from build123d import *

# Parameters (mm, degrees)
EXTRUDE019_DEPTH = 20
SKETCH022_R      = 2
EXTRUDE017_DEPTH = 7.5
FILLET008_R      = 2
SKETCH021_R      = 1
EXTRUDE016_DEPTH = 5
FILLET007_R      = 2
EXTRUDE018_DEPTH = 13
EXTRUDE007_DEPTH = 20
SKETCH008_R      = 1
EXTRUDE004_DEPTH = 5
FILLET001_R      = 2
SKETCH005_R      = 11.5
EXTRUDE003_DEPTH = 2.5
FILLET_R         = 1
SKETCH006_R      = 1.625
SKETCH006_R_2    = 5.532603
EXTRUDE002_DEPTH = 6
SKETCH009_R      = 2
EXTRUDE005_DEPTH = 7.5
FILLET002_R      = 2


with BuildPart() as extrude019:
    # Sketch024 (on Face5 of Cut001) → Extrude019 (new body, symmetric)
    with BuildSketch(Plane.XY.offset(6)):
        with BuildLine():
            ThreePointArc((18.40856, 16.235038), (15.499807, 18.5), (12.591346, 16.234663))
            ThreePointArc((12.10657, 15.857107), (12.413798, 15.962631), (12.591346, 16.234663))
            Line((12.10657, 15.857107), (12.10657, 10.857107))
            Line((12.10657, 10.857107), (18.905391, 10.857107))
            Line((18.905391, 15.85769), (18.905391, 10.857107))
            ThreePointArc((18.40856, 16.235038), (18.590902, 15.959369), (18.905391, 15.85769))
        make_face()
    extrude(amount=EXTRUDE019_DEPTH, both=True)


with BuildPart() as extrude019_1:
    # Extrude019 placement: moved
    add(extrude019.part.moved(Location((-31, 0, 10))))


with BuildPart() as fillet008:
    # Sketch022 (on Face2 of Cut001) → Extrude017 (new body)
    with BuildSketch(Plane(origin=(0, 20.857107, 0), x_dir=(-1, 0, 0), z_dir=(0, 1, 0))):
        with BuildLine():
            Line((-20.857107, 14.5), (-20.857107, 0))
            Line((-20.857107, 0), (-1.642893, 0))
            Line((-1.642893, 0), (-1.642893, 14.5))
            ThreePointArc((-1.642893, 14.5), (-2.375126, 16.267767), (-4.142893, 17))
            Line((-4.142893, 17), (-18.357107, 17))
            ThreePointArc((-18.357107, 17), (-20.124874, 16.267767), (-20.857107, 14.5))
        make_face()
        with Locations((-11.25, 11.5)):
            Circle(SKETCH022_R, mode=Mode.SUBTRACT)
    extrude(amount=EXTRUDE017_DEPTH)

    # Fillet008
    fillet008_edges = [fillet008.edges().sort_by_distance(p)[0] for p in [
        (20.124874, 28.357107, 16.267767),
    ]]
    fillet(fillet008_edges, radius=FILLET008_R)


with BuildPart() as fillet008_1:
    # Fillet008 placement: moved
    add(fillet008.part.moved(Location((-22.5, 0, 13))))


with BuildPart() as fillet007:
    # Sketch021 (on Face2 of Cut001) → Extrude016 (new body)
    with BuildSketch(Plane(origin=(0, 20.857107, 0), x_dir=(-1, 0, 0), z_dir=(0, 1, 0))):
        with BuildLine():
            Line((-20.857107, 14.5), (-20.857107, 0))
            Line((-20.857107, 0), (-1.642893, 0))
            Line((-1.642893, 0), (-1.642893, 14.5))
            ThreePointArc((-1.642893, 14.5), (-2.375126, 16.267767), (-4.142893, 17))
            Line((-4.142893, 17), (-18.357107, 17))
            ThreePointArc((-18.357107, 17), (-20.124874, 16.267767), (-20.857107, 14.5))
        make_face()
        with Locations((-11.25, 11.5)):
            Circle(SKETCH021_R, mode=Mode.SUBTRACT)
    extrude(amount=-EXTRUDE016_DEPTH)

    # Fillet007
    fillet007_edges = [fillet007.edges().sort_by_distance(p)[0] for p in [
        (20.124874, 15.857107, 16.267767),
    ]]
    fillet(fillet007_edges, radius=FILLET007_R)


with BuildPart() as fillet007_1:
    # Fillet007 placement: moved
    add(fillet007.part.moved(Location((-22.5, 0, 13))))


with BuildPart() as cut005:
    # Sketch023 (on Face5 of Fillet008) → Extrude018 (new body)
    with BuildSketch(Plane(origin=(-22.5, 0, 13), x_dir=(1, 0, 0), z_dir=(0, 0, -1))):
        with BuildLine():
            ThreePointArc((1.642893, -26.357107), (2.22868, -27.77132), (3.642893, -28.357107))
            Line((18.857107, -28.357107), (3.642893, -28.357107))
            ThreePointArc((18.857107, -28.357107), (20.27132, -27.77132), (20.857107, -26.357107))
            Line((20.857107, -17.857107), (20.857107, -26.357107))
            ThreePointArc((20.857107, -17.857107), (20.27132, -16.442893), (18.857107, -15.857107))
            Line((3.642893, -15.857107), (18.857107, -15.857107))
            ThreePointArc((3.642893, -15.857107), (2.22868, -16.442893), (1.642893, -17.857107))
            Line((1.642893, -26.357107), (1.642893, -17.857107))
        make_face()
    extrude(amount=EXTRUDE018_DEPTH)

    # Fusion006: union Fillet008, Fillet007
    add(fillet008_1.part)
    add(fillet007_1.part)

    # Cut005: cut Extrude019
    add(extrude019_1.part, mode=Mode.SUBTRACT)


with BuildPart() as extrude007:
    # Sketch011 (on Face5 of Cut001) → Extrude007 (new body, symmetric)
    with BuildSketch(Plane.XY.offset(6)):
        with BuildLine():
            ThreePointArc((18.40856, 16.235038), (15.499807, 18.5), (12.591346, 16.234663))
            ThreePointArc((12.10657, 15.857107), (12.413798, 15.962631), (12.591346, 16.234663))
            Line((12.10657, 15.857107), (12.10657, 10.857107))
            Line((12.10657, 10.857107), (18.905391, 10.857107))
            Line((18.905391, 15.85769), (18.905391, 10.857107))
            ThreePointArc((18.40856, 16.235038), (18.590902, 15.959369), (18.905391, 15.85769))
        make_face()
    extrude(amount=EXTRUDE007_DEPTH, both=True)


with BuildPart() as cut002:
    # Sketch008 (on Face2 of Cut001) → Extrude004 (new body)
    with BuildSketch(Plane(origin=(0, 20.857107, 0), x_dir=(-1, 0, 0), z_dir=(0, 1, 0))):
        with BuildLine():
            Line((-20.857107, 14.5), (-20.857107, 0))
            Line((-20.857107, 0), (-1.642893, 0))
            Line((-1.642893, 0), (-1.642893, 14.5))
            ThreePointArc((-1.642893, 14.5), (-2.375126, 16.267767), (-4.142893, 17))
            Line((-4.142893, 17), (-18.357107, 17))
            ThreePointArc((-18.357107, 17), (-20.124874, 16.267767), (-20.857107, 14.5))
        make_face()
        with Locations((-11.25, 11.5)):
            Circle(SKETCH008_R, mode=Mode.SUBTRACT)
    extrude(amount=-EXTRUDE004_DEPTH)

    # Fillet001
    fillet001_edges = [cut002.edges().sort_by_distance(p)[0] for p in [
        (20.124874, 15.857107, 16.267767),
    ]]
    fillet(fillet001_edges, radius=FILLET001_R)

    # Cut002: cut Extrude007
    add(extrude007.part, mode=Mode.SUBTRACT)


with BuildPart() as fillet_body:
    # Sketch005 (on Face5 of Part__Feature005) → Extrude003 (new body)
    with BuildSketch(Plane.XY):
        Circle(SKETCH005_R)
    extrude(amount=EXTRUDE003_DEPTH)

    # Fillet
    fillet_edges = [fillet_body.edges().sort_by_distance(p)[0] for p in [
        (-11.5, 0, 2.5),
    ]]
    fillet(fillet_edges, radius=FILLET_R)


with BuildPart() as bracket_base:
    # Sketch006 (on Face5 of Part__Feature005) → Extrude002 (new body)
    with BuildSketch(Plane.XY):
        with BuildLine():
            ThreePointArc((-18.357107, 20.857107), (-20.124874, 20.124874), (-20.857107, 18.357107))
            Line((-20.857107, -18.357107), (-20.857107, 18.357107))
            ThreePointArc((-20.857107, -18.357107), (-20.124874, -20.124874), (-18.357107, -20.857107))
            Line((18.357107, -20.857107), (-18.357107, -20.857107))
            ThreePointArc((18.357107, -20.857107), (20.124874, -20.124874), (20.857107, -18.357107))
            Line((20.857107, 18.357107), (20.857107, -18.357107))
            ThreePointArc((20.857107, 18.357107), (20.124874, 20.124874), (18.357107, 20.857107))
            Line((-18.357107, 20.857107), (18.357107, 20.857107))
        make_face()
        with Locations((-15.5, 15.5)):
            Circle(SKETCH006_R, mode=Mode.SUBTRACT)
        with Locations((15.5, 15.5)):
            Circle(SKETCH006_R, mode=Mode.SUBTRACT)
        with Locations((-15.5, -15.5)):
            Circle(SKETCH006_R, mode=Mode.SUBTRACT)
        with Locations((15.5, -15.5)):
            Circle(SKETCH006_R, mode=Mode.SUBTRACT)
        Circle(SKETCH006_R_2, mode=Mode.SUBTRACT)
    extrude(amount=EXTRUDE002_DEPTH)

    # Cut001: cut Fillet body
    add(fillet_body.part, mode=Mode.SUBTRACT)


with BuildPart() as driver_motor_bracket:
    # Sketch009 (on Face2 of Cut001) → Extrude005 (new body)
    with BuildSketch(Plane(origin=(0, 20.857107, 0), x_dir=(-1, 0, 0), z_dir=(0, 1, 0))):
        with BuildLine():
            Line((-20.857107, 14.5), (-20.857107, 0))
            Line((-20.857107, 0), (-1.642893, 0))
            Line((-1.642893, 0), (-1.642893, 14.5))
            ThreePointArc((-1.642893, 14.5), (-2.375126, 16.267767), (-4.142893, 17))
            Line((-4.142893, 17), (-18.357107, 17))
            ThreePointArc((-18.357107, 17), (-20.124874, 16.267767), (-20.857107, 14.5))
        make_face()
        with Locations((-11.25, 11.5)):
            Circle(SKETCH009_R, mode=Mode.SUBTRACT)
    extrude(amount=EXTRUDE005_DEPTH)

    # Fillet002
    fillet002_edges = [driver_motor_bracket.edges().sort_by_distance(p)[0] for p in [
        (20.124874, 28.357107, 16.267767),
    ]]
    fillet(fillet002_edges, radius=FILLET002_R)

    # Fusion007: union Cut005, Cut002, bracket base
    add(cut005.part)
    add(cut002.part)
    add(bracket_base.part)


solid = driver_motor_bracket.part
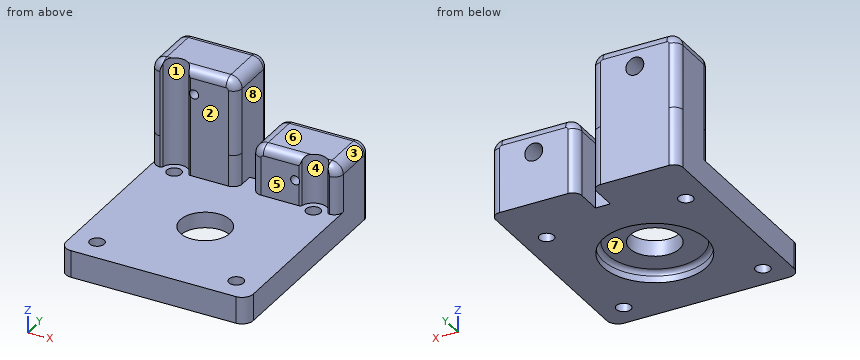
The listing builds one solid part. Answer for the finished solid, in the listing's coordinates (mm). Face numbers are marked on the shaded views. A direction names the side the tool comes from. Round coordinates to 2 decimals unless told otherwise and drop trailing zeros. Write each loop counter-clockwise with the first axis right and the second up, starting at its lowest first coordinate (ties: lowest second). Pieces come first, ordered by that corner, then holes. Notation, with made-up numbers: (10.25, 36) - (47.25, 36) arc R30 cw to (47.25, 58) - close; hole circle Ø7 at (-15.5, -40). An arc over 180 degrees is marked (long way). Use one line per item in the form item = value. Start each with the question number.
Item 1: A cutting plane is placed at B-B (x = 0). Write down the section's boundary in (y, z), plus the area to 3 significant figures.
Item 2: Find the intervals of material crossed by line 1 (X direction, y = 19.5, z = 7); line 2 (X direction, y = 0, z = 4); line 3 (Z direction, x = 11.25, y = 26.5), in increasing order. Write a range as [from, to].
Item 3: A cutting plane is placed at D-D (x = -15.5). Write down the section's boundary in (y, z) (3 decimals), plus the area to 3 significant figures.
Item 4: Determine the mould class of the marked faces 1, 2, 3 and 4 for opening direction X: +X half, -X half, draft (parallel to the pull), parting line (faces both ways), or undercut.
Item 5: A cutting plane is placed at A-A (y = 23). Write down the section's boundary in (x, z).
Item 6: A tool of negligible diameter and unlimited length cuts with its end or side. For the marked faces 5, 6, 7 and 8, from which of +Z, -Z, +X, -X, +Y, -Y can it reach the whole face along a straight path? Write none if from no direction.
Item 7: Flat-ended cylindrical pins translate along their axes: pin 1 Ø2 at (x, z) = (0, 3) entering from +Y; pin 2 Ø1.5 at (y, z) = (7, 7.5) entering from -X; pin 3 Ø7 at (x, y) = (14, 24) entering from +Z; pin 4 Ø6.5 at (x, y) = (-2.5, -1.5) entering from -Z. Find the tip coordinate at first contact, or state that the pin passes through.
The answers:
q1.outline = (-20.86, 0) - (-11.5, 0) - (-11.5, 1.5) arc R1 cw to (-10.5, 2.5) - (-5.53, 2.5) - (-5.53, 6) - (-20.86, 6) - close; (5.53, 2.5) - (10.5, 2.5) arc R1 cw to (11.5, 1.5) - (11.5, 0) - (20.86, 0) - (20.86, 6) - (5.53, 6) - close
q1.area = 154 mm^2
q2.line_1 = [-20.86, -1.64], [1.64, 20.86]
q2.line_2 = [-20.86, -5.53], [5.53, 20.86]
q2.line_3 = [0, 9.5], [13.5, 16.99]
q3.outline = (-20.857, 0) - (-17.125, 0) - (-17.125, 6) - (-20.857, 6) - close; (-13.875, 0) - (13.875, 0) - (13.875, 6) - (-13.875, 6) - close; (17.125, 0) - (28.357, 0) - (28.357, 28) arc R2 ccw to (26.357, 30) - (18.5, 30) - (18.5, 6) - (17.125, 6) - close
q3.area = 492 mm^2
q4.face_1 = undercut
q4.face_2 = draft
q4.face_3 = +X half
q4.face_4 = undercut
q5.outline = (-20.86, 0) - (-1.64, 0) - (-1.64, 27.5) arc R2.5 ccw to (-4.14, 30) - (-18.36, 30) arc R2.5 ccw to (-20.86, 27.5) - close; (1.64, 0) - (20.86, 0) - (20.86, 14.5) arc R2.5 ccw to (18.36, 17) - (4.14, 17) arc R2.5 ccw to (1.64, 14.5) - close; hole circle Ø4 at (-11.25, 24.5); hole circle Ø4 at (11.25, 11.5)
q6.face_5 = +Z, +X, -X, -Y
q6.face_6 = +Z, +X, +Y, -Y
q6.face_7 = -Z
q6.face_8 = +Z, +Y
q7.pin_1 = 20.86
q7.pin_2 = through
q7.pin_3 = 17
q7.pin_4 = 2.5
